Check sheet for the modelled part. Datum: model origin and axes. Units: mm. A direction names the side the tool comes from. Give positions to 0.01 mm unless a question says otherwise; leave off trailing zeros. Write each loop counter-clockwise with the first axis right and the second up, starting at its lowest first coordinate (ties: lowest second). Pieces come first, ordered by that corner, then holes. Notation, with made-up numbers: (64.25, 8.25) -> (109.25, 8.25) arc R18 ccw to (109.25, 30.25) -> close; hole circle Ø4 at (52.25, 8.25). An arc over 180 degrees is marked (long way). Return JSON: item names as keys, results as strings.
from build123d import *

# Parameters (mm, degrees)
SKETCH2_R          = 28.855655256
CUT_EXTRUDE1_DEPTH = 10


with BuildPart() as part:
    # Sketch1 → Revolve1 (revolve)
    with BuildSketch(Plane.XY, mode=Mode.PRIVATE) as revolve1_sk:
        Polygon((-9, 66.99759887), (-24, 66.99759887), (-24, 58.99759887), (-15.5, 58.99759887), (-15.5, 53.99759887), (-16, 53.99759887), (-16, 36.99759887), (-9, 36.99759887), align=None)
    revolve(revolve1_sk.sketch.rotate(Axis((0, 0, 0), (0, 1, 0)), 270), axis=Axis((0, 0, 0), (0, 1, 0)))

    # Sketch2 → Cut-Extrude1 (cut)
    with BuildSketch(Plane(origin=(0, 66.99759887, 0), x_dir=(-1, 0, 0), z_dir=(0, 1, 0))):
        Circle(SKETCH2_R)
        Polygon((0, -24), (20.784609691, -12), (20.784609691, 12), (0, 24), (-20.784609691, 12), (-20.784609691, -12), align=None, mode=Mode.SUBTRACT)
    extrude(amount=-CUT_EXTRUDE1_DEPTH, mode=Mode.SUBTRACT)


solid = part.part
(1) Cross-section at B-B on x = 2.5. Enter the section's corners in (y, z), then the cut area to 3 significant figures.
Reply:
{"outline": "(37, -15.8) -> (54, -15.8) -> (54, -15.3) -> (59, -15.3) -> (59, -22.56) -> (67, -22.56) -> (67, -8.65) -> (37, -8.65) -> close; (37, 8.65) -> (67, 8.65) -> (67, 22.56) -> (59, 22.56) -> (59, 15.3) -> (54, 15.3) -> (54, 15.8) -> (37, 15.8) -> close", "area": "532 mm^2"}
(2) Cross-section at C-C on y = 45. Enter the section's corners in (x, z).
Reply:
{"outline": "circle Ø32 at (0, 0); hole circle Ø18 at (0, 0)"}
(3) Set-up check for faces 1 (the flat face through (10.538, 63.054, -17.916)), 2 (the cylindrical face through (-15.368, 56.463, 2.018)): record each of +Z, -Z, +X, -X, +Y, -Y from which the full face is reachable in a straight line by a thin tool's end or side.
Reply:
{"face 1": "-Z, +X, +Y, -Y", "face 2": "none"}
(4) Release check for a two-part mould opening along Z. For faces 3 (the cylindrical face through (15.62, 45.38, 3.47)), 4 (the flat face through (-10.25, 63.05, -18.08)), 5 (the flat face through (-10.538, 63.054, 17.916)), 6 (the cylindrical face through (-2.703, 52.208, -8.584)) record: pulls with the +Z half, pulls with the -Z half, needs draft (parallel to the pull), parting line crosses it, or undercut.
Reply:
{"face 3": "parting line crosses it", "face 4": "pulls with the -Z half", "face 5": "pulls with the +Z half", "face 6": "undercut"}
(5) Depth check by flat-ended pin: pin 1 Ø2 at (x, y) = (11.5, 59) entering from +Z; pin 2 Ø1 at (x, y) = (-13, 50.5) entering from +Z; pin 3 Ø1 at (y, z) = (56, -4.5) entering from -X (3 decimals); pin 4 Ø9.5 at (x, z) = (0.5, -3.5) entering from +Y. Enter the tip coordinate at first touch or a pass-through.
Reply:
{"pin 1": "z = 17.94", "pin 2": "z = 9.99", "pin 3": "x = -14.975", "pin 4": "through"}
(6) Thickness scan on L1, parallel to X at y = 50, z = 0; L2, parallel to X at y = 55.5, z = 0; L3, parallel to Y at x = -10, z = -13.5. Record the ranges inside material, lowest first.
Reply:
{"L1": "-16 to -9, 9 to 16", "L2": "-15.5 to -9, 9 to 15.5", "L3": "59 to 67"}
(7) Cross-section at A-A on z = 0. Enter the section's corners in (x, y), then the cut area to 3 significant figures.
Reply:
{"outline": "(-20.78, 59) -> (-15.5, 59) -> (-15.5, 54) -> (-16, 54) -> (-16, 37) -> (-9, 37) -> (-9, 67) -> (-20.78, 67) -> close; (9, 37) -> (16, 37) -> (16, 54) -> (15.5, 54) -> (15.5, 59) -> (20.78, 59) -> (20.78, 67) -> (9, 67) -> close", "area": "492 mm^2"}
(8) Cross-section at D-D on x = -17. Enter the section's corners in (y, z), then the cut area to 3 significant figures.
Reply:
{"outline": "(59, -14.19) -> (67, -14.19) -> (67, 14.19) -> (59, 14.19) -> close", "area": "227 mm^2"}
